For this review, take the finished solid that the model builds, in its own axes (mm). Face numbers are marked on the shaded views. A direction names the side the tool comes from. Coordinates: 2 decimals unless noted, no trailing zeros. Write each loop counter-clockwise with the first axis right and the second up, starting at its lowest first coordinate (ties: lowest second). Pieces come first, ordered by that corner, then holes. Notation, with made-up numbers: (22.25, 88) - (28.25, 88) arc R22 ccw to (28.25, 116) - close; hole circle Ø2 at (84.5, 18.25). An arc over 180 degrees is marked (long way). Use one line per item in the form item = value. Start each with the question number.
1) We need section A-A (z = -152.4). Give the boundary of the cut face in (x, y), plus the area to 3 significant figures.
2) We need section B-B (y = 9). Give the boundary of the cut face in (x, z).
3) We need section D-D (z = -109). Give the boundary of the cut face in (x, y), plus the area to 3 significant figures.
4) We need section C-C (z = -88.9). Give the boundary of the cut face in (x, y), plus the area to 3 significant figures.
5) Tool access review of the marked faces 1 and 2: name each direction out of +Z, -Z, +X, -X, +Y, -Y from which nothing blocks a thin tool from reaching the whole face with its end or side.
6) For L1, parallel to Z at x = 19.05, y = 31; L2, parallel to Y at x = 9, z = -41; L3, parallel to X at y = 11.5, z = -152.4, list the stretches that pass through material, from the lowest coordinate up. Write a range as from..to.
7) Insertion check: P1, Ø6.5, axis at x = 72, y = 24.5, coming from the -Z side; P2, Ø1, axis at y = 43, z = -155, coming from the +X side; P3, Ø1.5, axis at x = 59.5, y = 33, coming from the +Z side; P4, Ø4, axis at y = 45.5, z = -21, coming from the -X side. Each pin has a flat end and moves straight along its axis. Give the tip position at first contact, or say it passes through.
```python
from build123d import *

# Parameters (mm, degrees)
BOSS_EXTRUDE1_DEPTH = 177.8
SKETCH8_R           = 10.16
CUT_EXTRUDE1_DEPTH  = 51.8
CHAMFER1_SIZE       = 5.08
SKETCH9_W           = 19.05
SKETCH9_H           = 76.2
CUT_EXTRUDE2_DEPTH  = 12.7
FILLET1_R           = 12.7
CUT_EXTRUDE3_DEPTH  = 31.75
FILLET2_R           = 12.7


with BuildPart() as part:
    # Sketch1 → Boss-Extrude1 (new body)
    with BuildSketch(Plane.XY):
        Polygon((0, 0), (0, 50.8), (38.1, 50.8), (76.2, 19.05), (76.2, 0), align=None)
    extrude(amount=-BOSS_EXTRUDE1_DEPTH)

    # Sketch8 → Cut-Extrude1 (cut, through all)
    with BuildSketch(Plane(origin=(0, 50.8, 0), x_dir=(1, 0, 0), z_dir=(0, 1, 0))):
        with Locations((19.05, 152.4)):
            Circle(SKETCH8_R)
    extrude(amount=-CUT_EXTRUDE1_DEPTH, mode=Mode.SUBTRACT)

    # Chamfer1
    chamfer1_edges = [part.edges().sort_by_distance(p)[0] for p in [
        (8.89, 50.8, -152.4),
    ]]
    chamfer(chamfer1_edges, length=CHAMFER1_SIZE)

    # Sketch9 → Cut-Extrude2 (cut)
    with BuildSketch(Plane(origin=(0, 50.8, 0), x_dir=(1, 0, 0), z_dir=(0, 1, 0))):
        with Locations((9.525, 38.1)):
            Rectangle(SKETCH9_W, SKETCH9_H)
    extrude(amount=-CUT_EXTRUDE2_DEPTH, mode=Mode.SUBTRACT)

    # Fillet1
    fillet1_edges = [part.edges().sort_by_distance(p)[0] for p in [
        (19.05, 44.45, -76.2),
    ]]
    fillet(fillet1_edges, radius=FILLET1_R)

    # Sketch10 → Cut-Extrude3 (cut)
    with BuildSketch(Plane(origin=(0, 50.8, 0), x_dir=(1, 0, 0), z_dir=(0, 1, 0))):
        with BuildLine():
            Line((76.2, 101.6), (60.198, 101.6))
            ThreePointArc((60.198, 101.6), (47.498, 88.9), (60.198, 76.2))
            Line((60.198, 76.2), (76.2, 76.2))
            Line((76.2, 76.2), (76.2, 101.6))
        make_face()
    extrude(amount=-CUT_EXTRUDE3_DEPTH, mode=Mode.SUBTRACT)

    # Fillet2
    fillet2_edges = [part.edges().sort_by_distance(p)[0] for p in [
        (0, 25.4, -177.8),
        (0, 19.05, 0),
        (76.2, 9.525, 0),
        (76.2, 9.525, -177.8),
    ]]
    fillet(fillet2_edges, radius=FILLET2_R)


solid = part.part
```
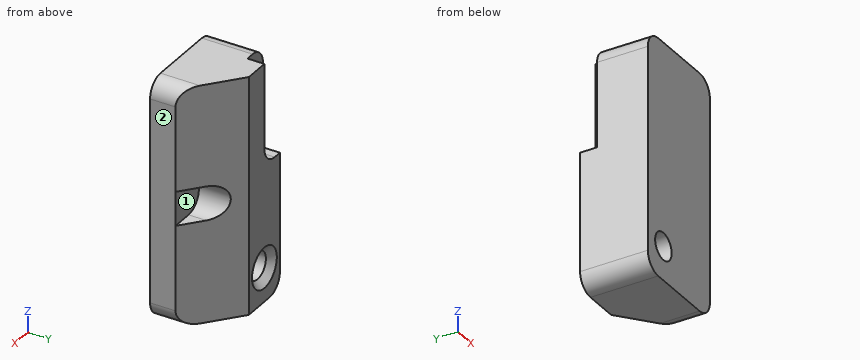
Determined:
q1.outline = (0, 0) - (8.89, 0) - (8.89, 45.72) - (3.81, 50.8) - (0, 50.8) - close; (29.21, 0) - (76.2, 0) - (76.2, 19.05) - (38.1, 50.8) - (34.29, 50.8) - (29.21, 45.72) - close
q1.area = 2,210 mm²
q2.outline = (0, -165.1) arc R12.7 ccw to (12.7, -177.8) - (63.5, -177.8) arc R12.7 ccw to (76.2, -165.1) - (76.2, -12.7) arc R12.7 ccw to (63.5, 0) - (12.7, 0) arc R12.7 ccw to (0, -12.7) - close; hole circle Ø20.32 at (19.05, -152.4)
q3.outline = (0, 0) - (76.2, 0) - (76.2, 19.05) - (38.1, 50.8) - (0, 50.8) - close
q3.area = 3,270 mm²
q4.outline = (0, 0) - (76.2, 0) - (76.2, 19.05) - (47.5, 19.05) - (47.5, 42.97) - (38.1, 50.8) - (0, 50.8) - close
q4.area = 2,920 mm²
q5.face_1 = +X, +Y
q5.face_2 = +Z, -Z, +X, +Y, -Y
q6.L1 = -177.8..-162.56, -142.24..0
q6.L2 = 0..38.1
q6.L3 = 0..8.89, 29.21..76.2
q7.P1 = -176.66
q7.P2 = 48.06
q7.P3 = 0
q7.P4 = 19.05
